Verification items for the finished model (mm, model axes). A direction names the side the tool comes from. Give positions to 0.01 mm unless a question says otherwise; leave off trailing zeros. Write each loop counter-clockwise with the first axis right and the second up, starting at its lowest first coordinate (ties: lowest second). Pieces come first, ordered by that corner, then holes. Notation, with made-up numbers: (61.25, -31) - (74.25, -31) arc R9 cw to (74.25, -26) - close; hole circle Ø7 at (42.25, 25). An arc over 180 degrees is marked (long way). Answer as a JSON object with one key per item and string values. Group by question number.
Item 1: Sectioned sample at D-D, the plane y = 0. Record the boundary of the cut face in (x, z), and give its area (3 significant figures).
Item 2: Go/stop test with flat-tipped pins: pin 1 (13.5 mm diameter, centred on x = -20, y = 0, fed in from +Z) (3 decimals); pin 2 (17 mm diameter, centred on x = -20, y = -40, fed in from -Z). Record where each tip stops, or that it passes through.
Item 3: Sectioned sample at B-B, the plane x = -20. Count the separate pieces of the cut face and the enclosed holes in it, and give its area (3 significant figures).
Item 4: Tool access check on faces 4 (the face through (-0.521, 28.966, 7.831)), 5 (the face through (-1.517, 18.166, 4.831)), 6 (the face through (-18.37, 47.32, 4.93)). Record the directions out of +Z, -Z, +X, -X, +Y, -Y that give a thin tool (end or side, any length) a straight path to the whole face; none if there is none.
Item 5: Sectioned sample at A-A, the plane y = 25. Record the boundary of the cut face in (x, z), and give its area (4 significant figures).
Item 6: Scan lines: line 1 along Y through (x, z) = (0, 4.3); line 2 along Y through (x, z) = (0, 9.15); line 3 along X through (y, z) = (-44.5, 3.5). Record each from-to range of solid material in increasing order. Write a range as [from, to].
Item 7: Draft check along X on faces 1 (the face through (15.155, -30.685, 3.451)), 2 (the face through (-35, 1, 5)), 3 (the face through (0, 60, 5)). Enter one of: +X half, -X half, draft (parallel to the pull), parting line (faces both ways), or undercut.
```python
from build123d import *

# Parameters (mm, degrees)
SKETCH_1_R          = 7.5
SKETCH_1_R_2        = 2.25
EXTRUDE_1_DEPTH     = 10
SKETCH_2_R          = 4
CUT_EXTRUDE_1_DEPTH = 4.4
SHELL_1_T           = -3


with BuildPart() as part:
    # 草图1 → 凸台-拉伸1 (new body)
    with BuildSketch(Plane.XY):
        with BuildLine():
            Line((-25, -60), (25, -60))
            ThreePointArc((25, -60), (32.071067812, -57.071067812), (35, -50))
            Line((35, -50), (35, 50))
            ThreePointArc((35, 50), (32.071067812, 57.071067812), (25, 60))
            Line((25, 60), (-25, 60))
            ThreePointArc((-25, 60), (-32.071067812, 57.071067812), (-35, 50))
            Line((-35, 50), (-35, -50))
            ThreePointArc((-35, -50), (-32.071067812, -57.071067812), (-25, -60))
        make_face()
        with Locations((20, 40)):
            Circle(SKETCH_1_R, mode=Mode.SUBTRACT)
        with Locations((20, 0)):
            Circle(SKETCH_1_R, mode=Mode.SUBTRACT)
        with Locations(Location((20, -40, 0), (0, 0, 180))):
            Circle(SKETCH_1_R, mode=Mode.SUBTRACT)
        with Locations((-20, -40)):
            Circle(SKETCH_1_R, mode=Mode.SUBTRACT)
        with Locations(Location((-20, 0, 0), (0, 0, 180))):
            Circle(SKETCH_1_R, mode=Mode.SUBTRACT)
        with Locations(Location((-20, 40, 0), (0, 0, 180))):
            Circle(SKETCH_1_R, mode=Mode.SUBTRACT)
        with Locations((0, 25)):
            Circle(SKETCH_1_R_2, mode=Mode.SUBTRACT)
        with Locations(Location((0, -25, 0), (0, 0, 180))):
            Circle(SKETCH_1_R_2, mode=Mode.SUBTRACT)
    extrude(amount=EXTRUDE_1_DEPTH)

    # 草图2 → 切除-拉伸1 (cut)
    with BuildSketch(Plane.XY.offset(10)):
        with Locations((0, 25)):
            Circle(SKETCH_2_R)
        with Locations((0, -25)):
            Circle(SKETCH_2_R)
    extrude(amount=-CUT_EXTRUDE_1_DEPTH, mode=Mode.SUBTRACT)

    # 抽壳1
    shell_1_openings = [part.faces().sort_by_distance(p)[0] for p in [
        (0, 0, 0),
    ]]
    offset(amount=SHELL_1_T, openings=shell_1_openings, kind=Kind.INTERSECTION)


solid = part.part
```
Geometry check:
{
 "1": {"outline": "(-35, 0) - (-32, 0) - (-32, 7) - (-30.5, 7) - (-30.5, 0) - (-27.5, 0) - (-27.5, 10) - (-35, 10) - close; (-12.5, 0) - (-9.5, 0) - (-9.5, 7) - (9.5, 7) - (9.5, 0) - (12.5, 0) - (12.5, 10) - (-12.5, 10) - close; (27.5, 0) - (30.5, 0) - (30.5, 7) - (32, 7) - (32, 0) - (35, 0) - (35, 10) - (27.5, 10) - close", "area": "246 mm^2"},
 "2": {"pin 1": "through", "pin 2": "z = 0"},
 "3": {"separate pieces": "4", "enclosed holes": "0", "area": "393 mm^2"},
 "4": {"face 4": "+Z", "face 5": "-Z", "face 6": "+Z, -Z"},
 "5": {"outline": "(-35, 0) - (-32, 0) - (-32, 7) - (-7, 7) - (-7, 2.6) - (-5.25, 2.6) - (-5.25, 0) - (-2.25, 0) - (-2.25, 5.6) - (-4, 5.6) - (-4, 10) - (-35, 10) - close; (2.25, 0) - (5.25, 0) - (5.25, 2.6) - (7, 2.6) - (7, 7) - (32, 7) - (32, 0) - (35, 0) - (35, 10) - (4, 10) - (4, 5.6) - (2.25, 5.6) - close", "area": "280.5 mm^2"},
 "6": {"line 1": "[-60, -57], [-32, -27.25], [-22.75, -18], [18, 22.75], [27.25, 32], [57, 60]", "line 2": "[-60, -29], [-21, 21], [29, 60]", "line 3": "[-35, -32], [-29.49, -26], [-14, -10.51], [10.51, 14], [26, 29.49], [32, 35]"},
 "7": {"face 1": "undercut", "face 2": "-X half", "face 3": "draft"}
}
